from build123d import *

# Parameters (mm, degrees)
F1_DEPTH = 12
F2_DEPTH = 4


with BuildPart() as f1:
    # F0 (on Front) → F1 (new body, symmetric)
    with BuildSketch(Plane.XZ):
        with BuildLine():
            ThreePointArc((-1.8533351034, 3.2312186547), (-2.2528950169, 2.2725457185), (-3.215001733, 1.8813263557))
            ThreePointArc((-3.215001733, 1.8813263557), (-3.7249912206, 0.0080874273), (-3.2231405801, -1.867348334))
            ThreePointArc((-3.2231405801, -1.867348334), (-2.2627416998, -2.2627416998), (-1.867348334, -3.2231405801))
            ThreePointArc((-1.867348334, -3.2231405801), (0, -3.725), (1.867348334, -3.2231405801))
            ThreePointArc((1.867348334, -3.2231405801), (2.2627416998, -2.2627416998), (3.2231405801, -1.867348334))
            ThreePointArc((3.2231405801, -1.867348334), (3.7249912206, 0.0080874273), (3.215001733, 1.8813263557))
            ThreePointArc((3.215001733, 1.8813263557), (2.2528950169, 2.2725457185), (1.8533351034, 3.2312186547))
            ThreePointArc((1.8533351034, 3.2312186547), (0, 3.725), (-1.8533351034, 3.2312186547))
        make_face()
        with BuildLine():
            ThreePointArc((-2.3419038887, 0.9), (-1.7775932123, 1.7844041548), (-0.9, 2.3592497012))
            ThreePointArc((-0.9, 2.3592497012), (0, 2.5269408414), (0.9, 2.3592497012))
            ThreePointArc((0.9, 2.3592497012), (1.7775932123, 1.7844041548), (2.3419038887, 0.9))
            ThreePointArc((2.3419038887, 0.9), (2.4594124113, 0.47098891), (2.499, 0.0279408414))
            ThreePointArc((2.499, 0.0279408414), (2.4539257567, -0.4445518891), (2.3203290273, -0.9))
            ThreePointArc((2.3203290273, -0.9), (1.75641402, -1.749701077), (0.9, -2.3033680185))
            ThreePointArc((0.9, -2.3033680185), (0, -2.4710591586), (-0.9, -2.3033680185))
            ThreePointArc((-0.9, -2.3033680185), (-1.75641402, -1.749701077), (-2.3203290273, -0.9))
            ThreePointArc((-2.3203290273, -0.9), (-2.4988205099, -0.0020101065), (-2.3419038887, 0.9))
        make_face(mode=Mode.SUBTRACT)
        with BuildLine():
            ThreePointArc((2.3419038887, 0.9), (1.7775932123, 1.7844041548), (0.9, 2.3592497012))
            Line((0.9, 2.3592497012), (0.9, 0.9))
            Line((0.9, 0.9), (2.3419038887, 0.9))
        make_face()
        with BuildLine():
            Line((-0.9, 0.9), (-0.9, 2.3592497012))
            ThreePointArc((-0.9, 2.3592497012), (-1.7775932123, 1.7844041548), (-2.3419038887, 0.9))
            Line((-2.3419038887, 0.9), (-0.9, 0.9))
        make_face()
        with BuildLine():
            ThreePointArc((0.9, -2.3033680185), (1.75641402, -1.749701077), (2.3203290273, -0.9))
            Line((2.3203290273, -0.9), (0.9, -0.9))
            Line((0.9, -0.9), (0.9, -2.3033680185))
        make_face()
        with BuildLine():
            Line((-0.9, -0.9), (-2.3203290273, -0.9))
            ThreePointArc((-2.3203290273, -0.9), (-1.75641402, -1.749701077), (-0.9, -2.3033680185))
            Line((-0.9, -2.3033680185), (-0.9, -0.9))
        make_face()
    extrude(amount=F1_DEPTH, both=True)

    # F0 (on Front) → F2 (join, symmetric)
    with BuildSketch(Plane.XZ):
        with BuildLine():
            ThreePointArc((0.9, 2.3592497012), (0, 2.5269408414), (-0.9, 2.3592497012))
            Line((-0.9, 2.3592497012), (-0.9, 0.9))
            Line((-0.9, 0.9), (-2.3419038887, 0.9))
            ThreePointArc((-2.3419038887, 0.9), (-2.4988205099, -0.0020101065), (-2.3203290273, -0.9))
            Line((-2.3203290273, -0.9), (-0.9, -0.9))
            Line((-0.9, -0.9), (-0.9, -2.3033680185))
            ThreePointArc((-0.9, -2.3033680185), (0, -2.4710591586), (0.9, -2.3033680185))
            Line((0.9, -2.3033680185), (0.9, -0.9))
            Line((0.9, -0.9), (2.3203290273, -0.9))
            ThreePointArc((2.3203290273, -0.9), (2.4539257567, -0.4445518891), (2.499, 0.0279408414))
            ThreePointArc((2.499, 0.0279408414), (2.4594124113, 0.47098891), (2.3419038887, 0.9))
            Line((2.3419038887, 0.9), (0.9, 0.9))
            Line((0.9, 0.9), (0.9, 2.3592497012))
        make_face()
    extrude(amount=F2_DEPTH, both=True)


solid = f1.part
Here's how the part is built. I have some questions about the finished solid (model axes, mm). A direction names the side the tool comes from. Round coordinates to 2 decimals unless told otherwise and drop trailing zeros. Write each loop counter-clockwise with the first axis right and the second up, starting at its lowest first coordinate (ties: lowest second). Pieces come first, ordered by that corner, then holes.
1. I need wall thicknesses on L1, parallel to Y at x = 0.5, z = 1.75; L2, parallel to X at y = -4.25, z = -0.75; L3, parallel to X at y = 5.5, z = 2. Which ranges of each line are inside material? Lowest first, please.
2. Will these pins go through, and if not, where does the flat tip stop? pin 1 Ø1.6 at (y, z) = (-7, 1.5) entering from -X; pin 2 Ø0.7 at (y, z) = (-9.5, -2) entering from -X; pin 3 Ø0.7 at (y, z) = (8, -1.5) entering from -X.
3. Suppose I cut it at D-D (y = 3.5). List the corners of the cut face in (x, z) for me (3 decimals).
4. Suppose I cut it at C-C (z = -0.5). List the corners of the cut face in (x, y) for me, and give its area (3 significant figures).
5. For faces 1 (the cylindrical face through (-0.013, -8.056, 2.527)), 2 (the flat face through (2, 8, -0.9)), which set-ups out of +Z, -Z, +X, -X, +Y, -Y let a thin tool reach every point of the face, with its end or its side?
6. Suppose I cut it at A-A (y = 6.25). List the corners of the cut face in (x, z) for me (3 decimals).
7. Suppose I cut it at B-B (x = 0). List the corners of the cut face in (y, z) for me (3 decimals).
8. If we mould it in two halves opening along Z, with no side actions, what happens to faces 3 (the flat face through (-2, 8, -0.9)), 4 (the cylindrical face through (3.725, -0.168, -0.019)), 5 (the flat face through (2, -12, -2)), 6 (the cylindrical face through (-2.5, 7.9, 0))? For each: released by +Z, released by -Z, zero draft, split by the parting line, or undercut.
Answer sheet:
1. L1: y = -4 to 4
1. L2: x = -3.65 to -2.37, 2.37 to 3.65
1. L3: x = -2.65 to -0.9, 0.9 to 2.65
2. pin 1: stops at x = -3.66
2. pin 2: stops at x = -3.34
2. pin 3: stops at x = -3.54
3. outline: (-3.223, -1.867) arc R1.35 cw to (-1.867, -3.223) arc R3.725 ccw to (1.867, -3.223) arc R1.35 cw to (3.223, -1.867) arc R3.725 ccw to (3.215, 1.881) arc R1.35 cw to (1.853, 3.231) arc R3.725 ccw to (-1.853, 3.231) arc R1.35 cw to (-3.215, 1.881) arc R3.725 ccw to start
4. outline: (-3.69, -12) - (-2.44, -12) - (-2.44, -4) - (2.44, -4) - (2.44, -12) - (3.69, -12) - (3.69, 12) - (2.44, 12) - (2.44, 4) - (-2.44, 4) - (-2.44, 12) - (-3.69, 12) - close
4. area: 99.0 mm2
5. face 1: -Y
5. face 2: +Y
6. outline: (-3.223, -1.867) arc R1.35 cw to (-1.867, -3.223) arc R3.725 ccw to (1.867, -3.223) arc R1.35 cw to (3.223, -1.867) arc R3.725 ccw to (3.215, 1.881) arc R1.35 cw to (1.853, 3.231) arc R3.725 ccw to (-1.853, 3.231) arc R1.35 cw to (-3.215, 1.881) arc R3.725 ccw to start; hole (-2.342, 0.9) arc R2.499 ccw to (-2.32, -0.9) - (-0.9, -0.9) - (-0.9, -2.303) arc R2.499 ccw to (0.9, -2.303) - (0.9, -0.9) - (2.32, -0.9) arc R2.499 ccw to (2.342, 0.9) - (0.9, 0.9) - (0.9, 2.359) arc R2.499 ccw to (-0.9, 2.359) - (-0.9, 0.9) - close
7. outline: (-12, -3.725) - (12, -3.725) - (12, -2.471) - (4, -2.471) - (4, 2.527) - (12, 2.527) - (12, 3.725) - (-12, 3.725) - (-12, 2.527) - (-4, 2.527) - (-4, -2.471) - (-12, -2.471) - close
8. face 3: undercut
8. face 4: split by the parting line
8. face 5: zero draft
8. face 6: undercut
